Verification items for this drawing (mm, ordinates from the low corner). A direction names the side the tool comes from. Give positions to 0.01 mm unless a question says otherwise; leave off trailing zeros. Loops run counter-clockwise (first coordinate to the right, second up) from the corner with the lowest first, then second, coordinate; pieces in that order, holes last. Notation, with made-up numbers: (68.5, 5) - (94.5, 5) arc R12 ccw to (94.5, 23) - close; hole circle Ø4 at (65.5, -11.5). An arc over 180 degrees is marked (long way). One line per question, with ' | ' between items. Start each with the question number.
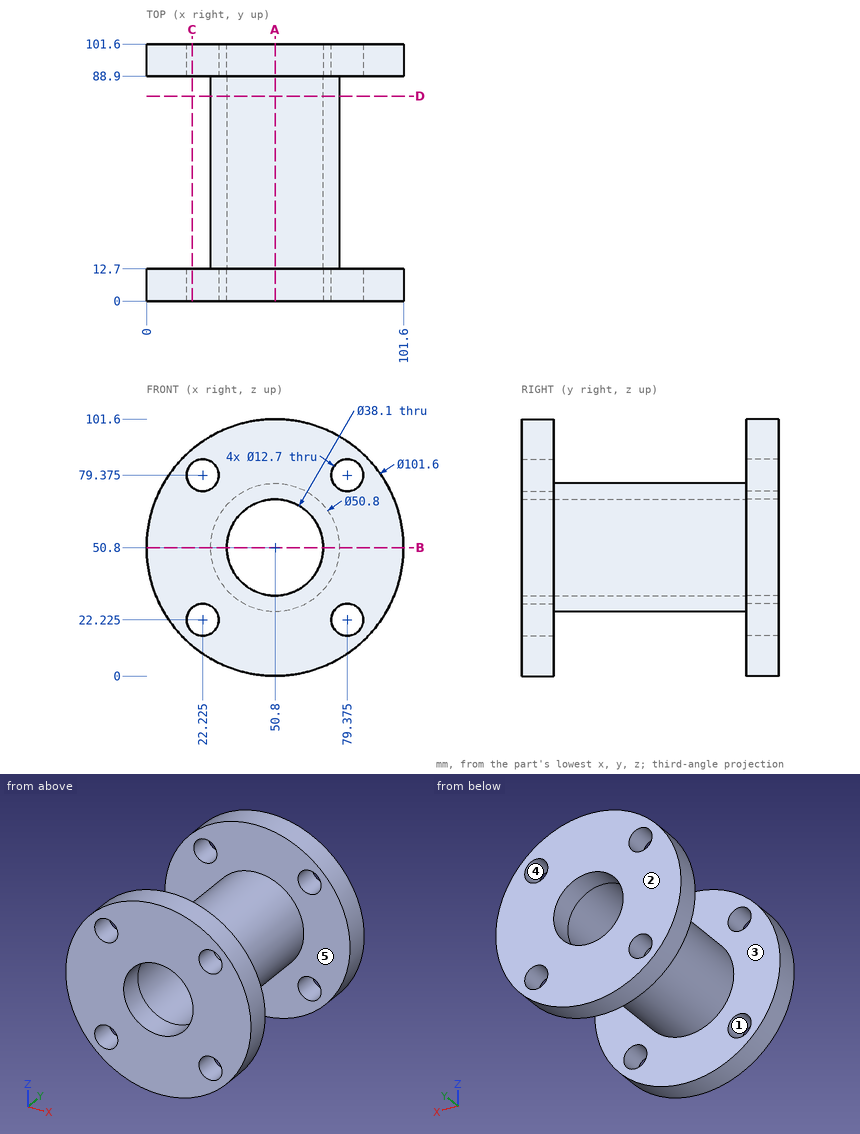
(1) Section check A-A, the plane x = 50.8. Record the boundary of the cut face in (y, z).
(2) Section check C-C, the plane x = 18. Record the boundary of the cut face in (y, z), and give its area (3 significant figures).
(3) Material ranges on line 1 (Y direction, x = 28, z = 66); line 2 (X direction, y = 97.5, z = 56.5); line 3 (X direction, y = 31, z = 68.5), recorded low to high.
(4) Tool access check on the marked faces 4 and 5. Record the directions out of +Z, -Z, +X, -X, +Y, -Y that give a thin tool (end or side, any length) a straight path to the whole face; none if there is none.
(5) Mould release check, pull along Y, two halves, no side actions. Record for the marked faces 1, 2 and 3: pulls with the +Y half, pulls with the -Y half, needs draft (parallel to the pull), parting line crosses it, or undercut.
(6) Section check D-D, the plane y = 81. Record the boundary of the cut face in (x, z).
(7) Depth check by flat-ended pin: pin 1 Ø2 at (x, y) = (68.5, 64.5) entering from -Z; pin 2 Ø23 at (x, z) = (50.8, 50.8) entering from +Y; pin 3 Ø10 at (y, z) = (45.5, 48) entering from +X; pin 4 Ø1.5 at (x, y) = (50, 47.5) entering from -Z. Enter the tip coordinate at first touch or a pass-through.
(8) Section check B-B, the plane z = 50.8. Record the boundary of the cut face in (x, y).
Numbers:
1) outline: (0, 0) - (12.7, 0) - (12.7, 25.4) - (88.9, 25.4) - (88.9, 0) - (101.6, 0) - (101.6, 31.75) - (0, 31.75) - close; (0, 69.85) - (101.6, 69.85) - (101.6, 101.6) - (88.9, 101.6) - (88.9, 76.2) - (12.7, 76.2) - (12.7, 101.6) - (0, 101.6) - close
2) outline: (0, 12.01) - (12.7, 12.01) - (12.7, 17.48) - (0, 17.48) - close; (0, 26.97) - (12.7, 26.97) - (12.7, 74.63) - (0, 74.63) - close; (0, 84.12) - (12.7, 84.12) - (12.7, 89.59) - (0, 89.59) - close; (88.9, 12.01) - (101.6, 12.01) - (101.6, 17.48) - (88.9, 17.48) - close; (88.9, 26.97) - (101.6, 26.97) - (101.6, 74.63) - (88.9, 74.63) - close; (88.9, 84.12) - (101.6, 84.12) - (101.6, 89.59) - (88.9, 89.59) - close | area: 1,490 mm^2
3) line 1: 0 to 12.7, 88.9 to 101.6 | line 2: 0.32 to 32.62, 68.98 to 101.28 | line 3: 32.58 to 43.76, 57.84 to 69.02
4) face 4: +Y, -Y | face 5: none
5) face 1: needs draft | face 2: pulls with the +Y half | face 3: undercut
6) outline: circle Ø50.8 at (50.8, 50.8); hole circle Ø38.1 at (50.8, 50.8)
7) pin 1: z = 31.66 | pin 2: through | pin 3: x = 76.2 | pin 4: z = 25.4
8) outline: (0, 0) - (31.75, 0) - (31.75, 101.6) - (0, 101.6) - (0, 88.9) - (25.4, 88.9) - (25.4, 12.7) - (0, 12.7) - close; (69.85, 0) - (101.6, 0) - (101.6, 12.7) - (76.2, 12.7) - (76.2, 88.9) - (101.6, 88.9) - (101.6, 101.6) - (69.85, 101.6) - close
